Build history of the part. All positions in model axes, mm. Coordinates: 2 decimals unless noted, no trailing zeros. Order: outer loops, then holes, each group sorted by start corner. A loop starts at its lowest first (then second) coordinate and runs counter-clockwise, first axis right, second up. Notation, with made-up numbers: (-39.5, 60.5) - (-0.5, 60.5) arc R4 cw to (-0.5, 66.5) - close; hole circle Ø5 at (-4, -31). An arc over 180 degrees is marked (long way). One line per item, written item: value.
from build123d import *

# Parameters (mm, degrees)
F3_R     = 77.5
F4_DEPTH = 225.001
F7_DEPTH = 500
F8_R     = 77.5
F9_DEPTH = 163.1971232988


with BuildPart() as f1:
    # F0 (on Front) → F1 (revolve)
    with BuildSketch(Plane.XZ):
        with BuildLine():
            Line((0, 0), (0, 200))
            ThreePointArc((0, 200), (-100, 100), (0, 0))
        make_face()
    revolve(axis=Axis((0, 0, 100), (0, 0, -1)))

    # F3 (on offset) → F4 (cut, through all)
    with BuildSketch(Plane.XY.offset(-25)):
        Circle(F3_R)
    extrude(amount=F4_DEPTH, mode=Mode.SUBTRACT)

    # F6 (on face) → F7 (join)
    with BuildSketch(Plane(origin=(0, 0, 0), x_dir=(-1, 0, 0), z_dir=(0, 1, 0))):
        with BuildLine():
            ThreePointArc((77.5, 36.8038767012), (100, 100), (77.5, 163.1961232988))
            Line((77.5, 163.1961232988), (0, 163.1961232988))
            Line((0, 163.1961232988), (0, 36.8038767012))
            Line((0, 36.8038767012), (77.5, 36.8038767012))
        make_face()
        with BuildLine():
            Line((0, 36.8038767012), (0, 163.1961232988))
            Line((0, 163.1961232988), (-77.5, 163.1961232988))
            ThreePointArc((-77.5, 163.1961232988), (-100, 100), (-77.5, 36.8038767012))
            Line((-77.5, 36.8038767012), (0, 36.8038767012))
        make_face()
    extrude(amount=F7_DEPTH)

    # F8 (on Top) → F9 (cut, through all)
    with BuildSketch(Plane.XY):
        Circle(F8_R)
    extrude(amount=F9_DEPTH, mode=Mode.SUBTRACT)


solid = f1.part
1. Band-saw the part on D-D, the plane y = 107. Give the cut face in (x, z).
Values found:
outline: (-77.5, 36.8) - (77.5, 36.8) arc R100 ccw to (77.5, 163.2) - (-77.5, 163.2) arc R100 ccw to start
2. Band-saw the part on A-A, the plane x = 0. Give the cut face in (y, z), and give its area (3 significant figures).
Values found:
outline: (-77.5, 36.8) - (-77.5, 163.2) arc R100 ccw to start; (77.5, 36.8) - (500, 36.8) - (500, 163.2) - (77.5, 163.2) - close
area: 55,300 mm2
3. Band-saw the part on C-C, the plane y = 39.5. Give the cut face in (x, z).
Values found:
outline: (-77.5, 36.8) - (-66.68, 36.8) - (-66.68, 163.2) - (-77.5, 163.2) arc R100 ccw to start; (66.68, 36.8) - (77.5, 36.8) arc R100 ccw to (77.5, 163.2) - (66.68, 163.2) - close
4. Band-saw the part on B-B, the plane z = 98. Give the cut face in (x, y), and give its area (3 significant figures).
Values found:
outline: (-99.98, 0) arc R99.98 ccw to (99.98, 0) - (99.98, 500) - (-99.98, 500) - close; hole circle Ø155 at (0, 0)
area: 96,800 mm2
5. Probe line 1 along Y through (x, z) = (0, 120.5); line 2 along Y through (x, z) = (40.5, 61); line 3 along X through (y, z) = (0, 102). List the from-to ranges inside material, lowest first.
Values found:
line 1: y = -97.88 to -77.5, 77.5 to 500
line 2: y = -82.7 to -66.08, 66.08 to 500
line 3: x = -99.98 to -77.5, 77.5 to 99.98
6. Flat gauge pins, fed straight in: P1, Ø5, axis at y = 4, z = 71, coming from the +X side; P2, Ø10, axis at y = 402.5, z = 88, coming from the -X side; P3, Ø4, axis at y = 7.5, z = 137, coming from the -X side (3 decimals). Where does each tip first touch, or does it go through?
Values found:
P1: stops at x = 96.42
P2: stops at x = -99.75
P3: stops at x = -93.675
7. Two-plate mould, pull along Y, no slides. Class faces 1 (the face through (-16.8, -75.657, 99.115)), 2 (the face through (-99.995, 246.5, 99.042)), 3 (the face through (1, 500, 101)): pulls with the +Y half, pulls with the -Y half, needs draft (parallel to the pull), parting line crosses it, or undercut.
Values found:
face 1: undercut
face 2: needs draft
face 3: pulls with the +Y half
